```python
from build123d import *

# Parameters (mm, degrees)
F3_D     = 3
F3_DEPTH = 5
F3_TIP   = 0.9012909285


with BuildPart() as f1:
    # F0 (on Front) → F1 (revolve)
    with BuildSketch(Plane.XZ):
        Polygon((-22.5, 20.6200371981), (-7, 20.6200371981), (-7, 36.6200371981), (-16.2, 36.6200371981), (-16.7, 37.1200371981), (-16.7, 38.6200371981), (-18.7, 38.6200371981), (-22.5, 23.6200371981), align=None)
    revolve(axis=Axis((0, 0, 28.6200371981), (0, 0, 1)))

    # F3
    with Locations(Plane(origin=(0, 0, 20.6200371981), x_dir=(1, 0, 0), z_dir=(0, 0, -1))):
        with Locations((-14, 0), (14, 0)):
            Hole(F3_D / 2, depth=F3_DEPTH)
            with Locations((0, 0, -(F3_DEPTH + F3_TIP / 2))):  # 118° drill point
                Cone(0, F3_D / 2, F3_TIP, mode=Mode.SUBTRACT)


solid = f1.part
```
The listing builds one solid part. Answer for the finished solid, in the listing's coordinates (mm). A direction names the side the tool comes from. Coordinates: 2 decimals unless noted, no trailing zeros. Loops run counter-clockwise (first coordinate to the right, second up) from the corner with the lowest first, then second, coordinate; pieces in that order, holes last. Notation, with made-up numbers: (44, -11.5) -> (61, -11.5) arc R6 ccw to (61, -4.5) -> close; hole circle Ø10 at (-28.75, 78). An arc over 180 degrees is marked (long way). Use one line per item in the form item = value. Start each with the question number.
Item 1: A tool of negligible diameter and unlimited length cuts with its end or side. For faces 4 (the face through (-12.5, -0.07, 23.16)), 5 (the face through (-6.466, 2.681, 28.732)), 6 (the face through (7, 3, 36.62)), from which of +Z, -Z, +X, -X, +Y, -Y can it reach the whole face along a straight path? Write none if from no direction.
Item 2: The part is cut by section A-A on x = 0. Determine the outline of the cut face in (y, z), then the cut area to 3 significant figures.
Item 3: Flat-ended cylindrical pins translate along their axes: pin 1 Ø4 at (x, y) = (-0.5, 11.5) entering from +Z; pin 2 Ø8 at (x, z) = (15.5, 34.5) entering from -Y; pin 3 Ø8 at (y, z) = (10.5, 37) entering from -X. Find the tip coordinate at first contact, or state that the pin passes through.
Item 4: Consider L1, parallel to Z at x = -6.5, y = 7; L2, parallel to Y at x = 6, z = 34.25; L3, parallel to X at y = 0, z = 38.15. Determine where each line is inside the solid, lowest interval first. Write a range as [from, to].
Item 5: The mould has two halves that part along Y. Classify faces 1 (the face through (-14.207, 0.159, 26.365)), 2 (the face through (-18.466, -5.815, 36.015)), 3 (the face through (-7.013, -15.324, 38.62)): released by +Y, released by -Y, zero draft, split by the parting line, or undercut.
Answer key:
q1.face_4 = -Z
q1.face_5 = +Z, -Z
q1.face_6 = +Z
q2.outline = (-22.5, 20.62) -> (-7, 20.62) -> (-7, 36.62) -> (-16.2, 36.62) -> (-16.7, 37.12) -> (-16.7, 38.62) -> (-18.7, 38.62) -> (-22.5, 23.62) -> close; (7, 20.62) -> (22.5, 20.62) -> (22.5, 23.62) -> (18.7, 38.62) -> (16.7, 38.62) -> (16.7, 37.12) -> (16.2, 36.62) -> (7, 36.62) -> close
q2.area = 462 mm2
q3.pin_1 = 36.62
q3.pin_2 = -16.31
q3.pin_3 = -18.32
q4.L1 = [20.62, 36.62]
q4.L2 = [-18.88, -3.61], [3.61, 18.88]
q4.L3 = [-18.82, -16.7], [16.7, 18.82]
q5.face_1 = undercut
q5.face_2 = split by the parting line
q5.face_3 = zero draft
